```python
from build123d import *

# Parameters (mm, degrees)
SKETCH2_W           = 50
SKETCH2_H           = 110
SKETCH2_R           = 15
BOSS_EXTRUDE1_DEPTH = 20
SKETCH3_R           = 32.015621187
BOSS_EXTRUDE2_DEPTH = 20


with BuildPart() as part:
    # Sketch2 → Boss-Extrude1 (new, symmetric)
    with BuildSketch(Plane.XY):
        with Locations((0, -25)):
            Rectangle(SKETCH2_W, SKETCH2_H)
        Circle(SKETCH2_R, mode=Mode.SUBTRACT)
    extrude(amount=BOSS_EXTRUDE1_DEPTH, both=True)

    # Sketch3 → Boss-Extrude2 (add)
    with BuildSketch(Plane.XZ.offset(80)):
        with Locations(Location((0, 0, 0), (0, 0, 270))):
            Circle(SKETCH3_R)
    extrude(amount=-BOSS_EXTRUDE2_DEPTH)


solid = part.part
```
The model under review builds one solid part; all positions refer to its coordinate system, in mm. A direction names the side the tool comes from. Coordinates: 2 decimals unless noted, no trailing zeros. Write each loop counter-clockwise with the first axis right and the second up, starting at its lowest first coordinate (ties: lowest second). Pieces come first, ordered by that corner, then holes. Notation, with made-up numbers: (-10.5, 62.25) -> (41.5, 62.25) arc R30 cw to (41.5, 88.25) -> close; hole circle Ø9 at (-8, 62). An arc over 180 degrees is marked (long way). One line per item, written item: value. Start each with the question number.
Q1. The part is to be moulded in two halves that separate along Y. For faces 1 (the face through (-25, -16, 0)), 2 (the face through (-14.985, 0.66, -0.28)), 3 (the face through (-28, -60, 0)), say which applies: +Y half, -Y half, draft (parallel to the pull), parting line (faces both ways), or undercut.
Q2. To check wall thickness, follow probe 1 along Y at (x, z) = (0, -10.5); probe 2 along Z at (x, y) = (11.5, 15.5); probe 3 along Y at (x, z) = (-5, 17.5). State the ranges of each line that lie inside material, in increasing order.
Q3. Add section A-A, the plane y = 0. Give the boundary of the cut face in (x, z).
Q4. Clearance check with flat-ended pins moving along their axes: P1, Ø5.5, axis at x = -30, z = -4.5, coming from the +Y side; P2, Ø25, axis at x = 5.5, y = -28, coming from the +Z side; P3, Ø12, axis at y = -2.5, z = -0.5, coming from the -X side. State where each tip first meets the part, or that it passes through.
Q5. Add section C-C, the plane z = 0. Give the boundary of the cut face in (x, y).
Q6. Add section B-B, the plane x = 0. Give the boundary of the cut face in (y, z), then the cut area to 3 significant figures.
Q7. Add section D-D, the plane x = 20. Give the boundary of the cut face in (y, z).
Q8. For faces 4 (the face through (-6, -14, 20)), 5 (the face through (28, -60, 0)), 6 (the face through (0, 30, 0)), 7 (the face through (0, -80, 0)), 8 (the face through (0, -60, -25)), list the 3-axis set-ups (+Z, -Z, +X, -X, +Y, -Y) from which the entire face can be reached by the end or side of a thin tool; tool diameter is ignored.
Response:
1. face 1: draft
1. face 2: undercut
1. face 3: +Y half
2. probe 1: -80 to -15, 15 to 30
2. probe 2: -20 to 20
2. probe 3: -80 to -14.14, 14.14 to 30
3. outline: (-25, -20) -> (-15, -20) -> (-15, 20) -> (-25, 20) -> close; (15, -20) -> (25, -20) -> (25, 20) -> (15, 20) -> close
4. P1: y = -60
4. P2: z = 20
4. P3: x = -25
5. outline: (-32.02, -80) -> (32.02, -80) -> (32.02, -60) -> (25, -60) -> (25, 30) -> (-25, 30) -> (-25, -60) -> (-32.02, -60) -> close; hole circle Ø30 at (0, 0)
6. outline: (-80, -32.02) -> (-60, -32.02) -> (-60, -20) -> (-15, -20) -> (-15, 20) -> (-60, 20) -> (-60, 32.02) -> (-80, 32.02) -> close; (15, -20) -> (30, -20) -> (30, 20) -> (15, 20) -> close
6. area: 3,680 mm²
7. outline: (-80, -25) -> (-60, -25) -> (-60, -20) -> (30, -20) -> (30, 20) -> (-60, 20) -> (-60, 25) -> (-80, 25) -> close
8. face 4: +Z, +X, -X, +Y
8. face 5: +Z, -Z, +X, +Y
8. face 6: +Z, -Z, +X, -X, +Y
8. face 7: +Z, -Z, +X, -X, -Y
8. face 8: -Z, +X, -X, +Y
